Here's how the part is built. I have some questions about the finished solid (model axes, mm). Face numbers are marked on the shaded views. Round coordinates to 2 decimals unless told otherwise and drop trailing zeros. Write each loop counter-clockwise with the first axis right and the second up, starting at its lowest first coordinate (ties: lowest second). Pieces come first, ordered by that corner, then holes. Notation, with made-up numbers: (-14.75, -9.5) -> (43.25, -9.5) arc R7 ccw to (43.25, -4.5) -> close; hole circle Ø3 at (5.5, 67.25). An arc over 180 degrees is marked (long way). Answer as CSV lines item,"result".
from build123d import *

# Parameters (mm, degrees)
F0_R     = 12.7
F1_DEPTH = 50.8


# Not quite as in the source:
# - the program builds the solid bodies; features that only make, move or delete a surface that nothing else refers to are left out


with BuildPart() as f1:
    # F0 (on Top) → F1 (new body)
    with BuildSketch(Plane.XY):
        with BuildLine():
            ThreePointArc((3.81, -37.9090213538), (28.2557162358, -25.5582569828), (38.1, 0))
            ThreePointArc((38.1, 0), (28.2557162358, 25.5582569828), (3.81, 37.9090213538))
            ThreePointArc((3.81, 37.9090213538), (-38.1, 0), (3.81, -37.9090213538))
        make_face()
        Circle(F0_R, mode=Mode.SUBTRACT)
        with BuildLine():
            ThreePointArc((3.81, 37.9090213538), (28.2557162358, 25.5582569828), (38.1, 0))
            ThreePointArc((38.1, 0), (28.2557162358, -25.5582569828), (3.81, -37.9090213538))
            Line((3.81, -37.9090213538), (129.54, -25.2726809025))
            ThreePointArc((129.54, -25.2726809025), (101.6, 0), (129.54, 25.2726809025))
            Line((129.54, 25.2726809025), (3.81, 37.9090213538))
        make_face()
        with BuildLine():
            ThreePointArc((152.4, 0), (145.8371441572, 17.0388379885), (129.54, 25.2726809025))
            ThreePointArc((129.54, 25.2726809025), (101.6, 0), (129.54, -25.2726809025))
            ThreePointArc((129.54, -25.2726809025), (145.8371441572, -17.0388379885), (152.4, 0))
        make_face()
        with Locations((127, 0)):
            Circle(F0_R, mode=Mode.SUBTRACT)
    extrude(amount=F1_DEPTH)


solid = f1.part
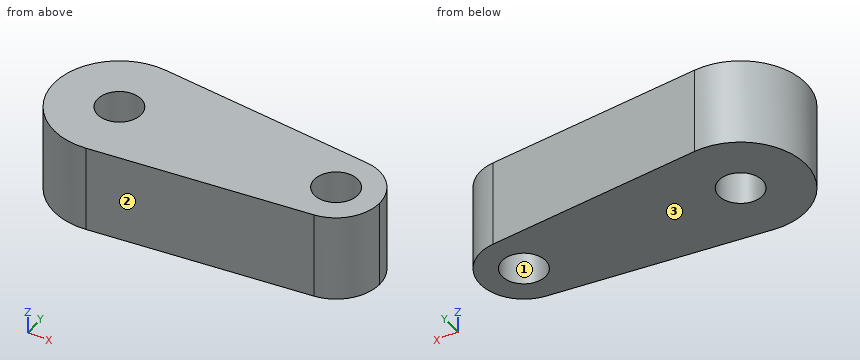
Item 1: If we mould it in two halves opening along X, with no side actions, what happens to the marked faces 1, 2 and 3? For each: pulls with the +X half, pulls with the -X half, needs draft (parallel to the pull), parting line crosses it, or undercut.
Results found:
face 1,"undercut"
face 2,"pulls with the +X half"
face 3,"needs draft"
Item 2: Will these pins go through, and if not, where does the flat tip stop? pin 1 (8 mm diameter, centred on y = -15.5, z = 13.5, fed in from -X); pin 2 (1 mm diameter, centred on y = 13.5, z = 7.5, fed in from -X); pin 3 (12 mm diameter, centred on y = 1.5, z = 19.5, fed in from -X); pin 4 (6 mm diameter, centred on x = -6.5, z = 10.5, fed in from -Y).
Results found:
pin 1,"stops at x = -36.32"
pin 2,"stops at x = -35.81"
pin 3,"stops at x = -38.1"
pin 4,"stops at y = -37.94"
Item 3: Suppose I cut it at C-C, the plane y = -5. List the corners of the cut face in (x, z) for me.
Results found:
outline,"(-37.77, 0) -> (-11.67, 0) -> (-11.67, 50.8) -> (-37.77, 50.8) -> close; (11.67, 0) -> (115.33, 0) -> (115.33, 50.8) -> (11.67, 50.8) -> close; (138.67, 0) -> (151.9, 0) -> (151.9, 50.8) -> (138.67, 50.8) -> close"
Item 4: Suppose I cut it at D-D, the plane x = 127. List the corners of the cut face in (y, z) for me.
Results found:
outline,"(-25.53, 0) -> (-12.7, 0) -> (-12.7, 50.8) -> (-25.53, 50.8) -> close; (12.7, 0) -> (25.53, 0) -> (25.53, 50.8) -> (12.7, 50.8) -> close"
Item 5: I need wall thicknesses on L1, parallel to Y at x = 0, z = 25; L2, parallel to X at y = 8, z = 14.5; L3, parallel to X at y = 5, z = 38. Which ranges of each line are inside material? Lowest first, please.
Results found:
L1,"y = -38.1 to -12.7, 12.7 to 38.1"
L2,"x = -37.25 to -9.86, 9.86 to 117.14, 136.86 to 151.11"
L3,"x = -37.77 to -11.67, 11.67 to 115.33, 138.67 to 151.9"
Item 6: Suppose I cut it at A-A, the plane x = 0. List the corners of the cut face in (y, z) for me, then the cut area to 3 significant figures.
Results found:
outline,"(-38.1, 0) -> (-12.7, 0) -> (-12.7, 50.8) -> (-38.1, 50.8) -> close; (12.7, 0) -> (38.1, 0) -> (38.1, 50.8) -> (12.7, 50.8) -> close"
area,"2,580 mm²"
Item 7: Suppose I cut it at B-B, the plane z = 34.5. List the corners of the cut face in (x, y) for me.
Results found:
outline,"(3.81, -37.91) -> (129.54, -25.27) arc R25.4 ccw to (129.54, 25.27) -> (3.81, 37.91) arc R38.1 ccw (long way) to start; hole circle Ø25.4 at (0, 0); hole circle Ø25.4 at (127, 0)"
